from build123d import *

# Parameters (mm, degrees)
SKETCH_1_W          = 28
SKETCH_1_H          = 20
SKETCH_1_R          = 1
EXTRUDE_1_DEPTH     = 3
CUT_EXTRUDE_1_DEPTH = 4
SKETCH_3_W          = 17.35128085
SKETCH_3_H          = 5.450829119
SKETCH_3_W_2        = 17.701224177
SKETCH_3_H_2        = 5.124932949
EXTRUDE_2_DEPTH     = 3


with BuildPart() as part:
    # 草图1 → 凸台-拉伸1 (new body)
    with BuildSketch(Plane.XY):
        Rectangle(SKETCH_1_W, SKETCH_1_H)
        with Locations((8, 4.75)):
            Circle(SKETCH_1_R, mode=Mode.SUBTRACT)
        with Locations((8, -4.75)):
            Circle(SKETCH_1_R, mode=Mode.SUBTRACT)
        with BuildLine():
            Line((-11, 6.25), (1, 6.25))
            ThreePointArc((1, 6.25), (2.5, 4.75), (1, 3.25))
            Line((1, 3.25), (-11, 3.25))
            ThreePointArc((-11, 3.25), (-12.5, 4.75), (-11, 6.25))
        make_face(mode=Mode.SUBTRACT)
        with BuildLine():
            Line((-11, -6.25), (1, -6.25))
            ThreePointArc((1, -6.25), (2.5, -4.75), (1, -3.25))
            Line((1, -3.25), (-11, -3.25))
            ThreePointArc((-11, -3.25), (-12.5, -4.75), (-11, -6.25))
        make_face(mode=Mode.SUBTRACT)
    extrude(amount=EXTRUDE_1_DEPTH)

    # 草图2 → 切除-拉伸1 (cut, through all)
    with BuildSketch(Plane.XY.offset(3)):
        with BuildLine():
            Line((1, -1.5), (-11, -1.5))
            ThreePointArc((-11, -1.5), (-12.5, 0), (-11, 1.5))
            Line((-11, 1.5), (1, 1.5))
            ThreePointArc((1, 1.5), (2.5, 0), (1, -1.5))
        make_face()
    extrude(amount=-CUT_EXTRUDE_1_DEPTH, mode=Mode.SUBTRACT)

    # 草图3 → 凸台-拉伸2 (add)
    with BuildSketch(Plane.XY.offset(3)):
        with Locations((-4.556899514, 5.212806564)):
            Rectangle(SKETCH_3_W, SKETCH_3_H)
        with Locations((-4.381927851, -5.15844561)):
            Rectangle(SKETCH_3_W_2, SKETCH_3_H_2)
    extrude(amount=-EXTRUDE_2_DEPTH)


solid = part.part
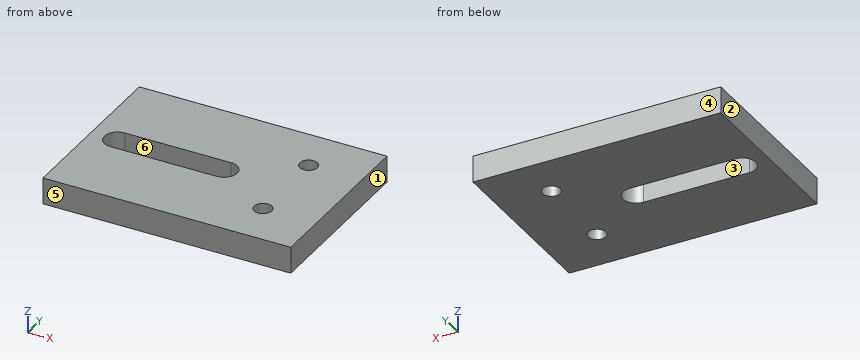
Part model, mm, in its own coordinate system. Face numbers are marked on the shaded views. A direction names the side the tool comes from. Coordinates: 2 decimals unless noted, no trailing zeros. Loops run counter-clockwise (first coordinate to the right, second up) from the corner with the lowest first, then second, coordinate; pieces in that order, holes last. Notation, with made-up numbers: (64.25, 41) - (90.25, 41) arc R20 ccw to (90.25, 54) - close; hole circle Ø6 at (48, 58). An arc over 180 degrees is marked (long way). Write each question's results on one line, items separated by ' | '. Start each with the question number.
Q1. Drop a flat-ended pin along its axis: pin 1 Ø1.8 at (x, y) = (8, -4.75) entering from +Z. Give the stop position or say it passes through.
Q2. Slice it at C-C on z = 1. Give the cut face in (x, y), and give its area (3 significant figures).
Q3. Two-plate mould, pull along X, no slides. Class the marked faces 1, 2, 3 and 4: +X half, -X half, draft (parallel to the pull), parting line (faces both ways), or undercut.
Q4. Slice it at B-B on x = 8. Give the cut face in (y, z), and give its area (3 significant figures).
Q5. Slice it at D-D on x = -8.5. Give the cut face in (y, z).
Q6. Slice it at A-A on y = -4.75. Give the cut face in (x, z), and give its area (3 significant figures).
Q7. Probe line 1 along Y through (x, z) = (8, 0.7); line 2 along Y through (x, z) = (-2.5, 2.7); line 3 along X through (y, z) = (5, 0.45). List the from-to ranges inside material, lowest first.
Q8. Which spindle directions (+Z, -Z, +X, -X, +Y, -Y) get a long thin tool onto all of the face, cutting with end or side? Do the marked faces 5 and 6. Say none if no direction does.
Answer:
1) pin 1: passes through
2) outline: (-14, -10) - (14, -10) - (14, 10) - (-14, 10) - close; hole (-11, -1.5) - (1, -1.5) arc R1.5 ccw to (1, 1.5) - (-11, 1.5) arc R1.5 ccw to start; hole circle Ø2 at (8, -4.75); hole circle Ø2 at (8, 4.75) | area: 511 mm2
3) face 1: +X half | face 2: -X half | face 3: undercut | face 4: draft
4) outline: (-10, 0) - (-5.75, 0) - (-5.75, 3) - (-10, 3) - close; (-3.75, 0) - (3.75, 0) - (3.75, 3) - (-3.75, 3) - close; (5.75, 0) - (10, 0) - (10, 3) - (5.75, 3) - close | area: 48.0 mm2
5) outline: (-10, 0) - (-1.5, 0) - (-1.5, 3) - (-10, 3) - close; (1.5, 0) - (10, 0) - (10, 3) - (1.5, 3) - close
6) outline: (-14, 0) - (7, 0) - (7, 3) - (-14, 3) - close; (9, 0) - (14, 0) - (14, 3) - (9, 3) - close | area: 78.0 mm2
7) line 1: y = -10 to -5.75, -3.75 to 3.75, 5.75 to 10 | line 2: y = -10 to -1.5, 1.5 to 10 | line 3: x = -14 to 7.03, 8.97 to 14
8) face 5: +Z, -Z, +X, -X, -Y | face 6: +Z, -Z
